The model under review builds one solid part; all positions refer to its coordinate system, in mm. Coordinates: 2 decimals unless noted, no trailing zeros. Write each loop counter-clockwise with the first axis right and the second up, starting at its lowest first coordinate (ties: lowest second). Pieces come first, ordered by that corner, then holes.
1) Add section A-A, the plane y = 19. State the section outline as (x, z) points.
2) Add section B-B, the plane z = 1.3. State the section outline as (x, y) points.
3) For line 1 (Y direction, x = -10, z = 0.7); line 2 (X direction, y = 19, z = 1.35); line 3 (X direction, y = -6, z = 1.05), list the stretches that pass through material, from the lowest coordinate up.
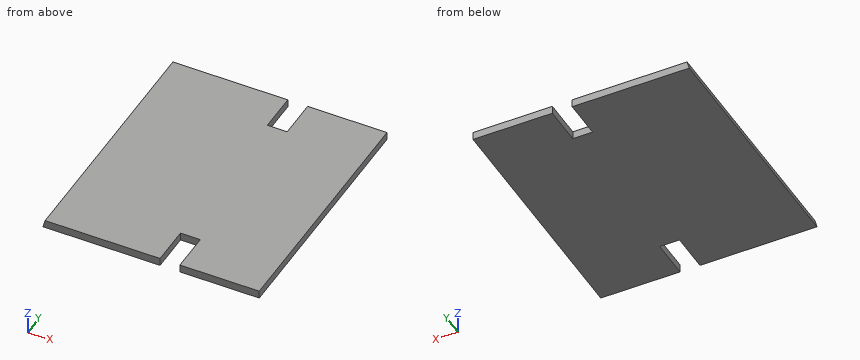
Autodesk Inventor part; units mm, degrees
ref_plane "YZ Plane" through (0, 0, 0) normal (1, 0, 0) x (0, 1, 0)
ref_plane "XZ Plane" through (0, 0, 0) normal (0, 1, 0) x (-1, 0, 0)
ref_plane "XY Plane" through (0, 0, 0) normal (0, 0, 1) x (1, 0, 0)
sketch "Szkic1" plane through (0, 0, 0) normal (0, 0, 1) x (1, 0, 0)
  line L0 (-43, 25) -> (-7, 25)
  line L1 (-7, 25) -> (-7, 11)
  line L2 (-7, 11) -> (7, 11)
  line L3 (7, 11) -> (7, -11)
  line L4 (7, -11) -> (-7, -11)
  line L5 (-7, -11) -> (-7, -25)
  line L6 (-7, -25) -> (-43, -25)
  line L7 (-7, -11) -> (7, -11)
  line L8 (7, -11) -> (7, -25)
  line L9 (7, -25) -> (-7, -25)
  line L10 (-7, -25) -> (-7, -11)
  line L11 (-7, 11) -> (7, 11)
  line L12 (7, 11) -> (7, 25)
  line L13 (7, 25) -> (-7, 25)
  line L14 (-7, 25) -> (-7, 11)
  line L15 (-43, -25) -> (-43, 25)
  point P0 (0, 0)
  point P1 (7, 11)
  point P2 (7, 11)
extrude "Wyciągnięcie proste1" add sketch "Szkic1" along normal blind 1.6
ref_plane "Płaszczyzna konstrukcyjna1" through (-17.9997, 25, -4.7) normal (0, 1, 0) x (0, 0, 1)
sketch "Szkic3" plane through (0, 0, 1.6) normal (0, 0, 1) x (1, 0, 0)
  line L0 (-43, -25) -> (7, -25)
  line L1 (7, -25) -> (7, 25)
  line L2 (7, 25) -> (-43, 25)
  line L3 (-13, -25) -> (-9, -25)
  line L4 (-9, -25) -> (-9, -17)
  line L5 (-9, -17) -> (-13, -17)
  line L6 (-13, -17) -> (-13, -25)
  line L7 (7, 25) -> (-40.2936, 25)
  line L8 (-9, 25) -> (-13, 25)
  line L9 (-13, 25) -> (-13, 17)
  line L10 (-13, 17) -> (-9, 17)
  line L11 (-9, 17) -> (-9, 25)
  line L12 (-43, 25) -> (-43, -25)
  point P0 (0, 0)
  point P1 (-35.2314, 25)
  point P2 (-35.7424, 25)
  point P3 (-11, 25)
  dimension "d4" = 16
  dimension "d5" = 16
  dimension "d6" = 8
  dimension "d7" = 8
  dimension "d8" = 4
  dimension "d9" = 4
extrude "Wyciągnięcie proste3" cut sketch "Szkic3" against normal through all contours L6 L5 L4 L0 | L2 L11 L10 L9
sketch "Szkic4" plane through (-40.2936, 25, 1.6) normal (0, 1, 0) x (1, 0, 0)
  line L0 (4.9241, -3) -> (-0.6358, 17.75)
  line L1 (-0.6358, 17.75) -> (-2.7064, 17.75)
  line L2 (-2.7064, 17.75) -> (2.8536, -3)
  line L3 (2.8536, -3) -> (4.9241, -3)
  line L4 (27.2936, 0) -> (27.2936, 1.6)
  line L5 (47.2936, 1.6) -> (31.2936, 1.6)
  line L6 (27.2936, 0) -> (-2.7064, 0)
  line L7 (27.2936, 1.6) -> (-2.7064, 1.6)
  line L8 (-2.7064, 1.6) -> (-2.7064, 0)
  line L9 (31.2936, 1.6) -> (31.2936, 0)
  line L10 (47.2936, 0) -> (31.2936, 0)
  line L11 (47.2936, 1.6) -> (47.2936, 0)
  point P0 (40.2936, 1.6)
  point P1 (3.6916, 1.6)
  point P2 (4.1203, 0)
extrude "Wyciągnięcie proste4" cut sketch "Szkic4" against normal through all contours L6 L2 L7 L0 | L6 L8 L7 L2
properties part number "pcb"
Geometry results:
1. outline: (-36.6, 0) - (-13, 0) - (-13, 1.6) - (-36.17, 1.6) - close; (-9, 0) - (7, 0) - (7, 1.6) - (-9, 1.6) - close
2. outline: (-36.25, -25) - (-13, -25) - (-13, -17) - (-9, -17) - (-9, -25) - (7, -25) - (7, 25) - (-9, 25) - (-9, 17) - (-13, 17) - (-13, 25) - (-36.25, 25) - close
3. line 1: y = -17 to 17
3. line 2: x = -36.24 to -13, -9 to 7
3. line 3: x = -36.32 to 7
